```python
from build123d import *

# Parameters (mm, degrees)
F1_W         = 152.4
F1_H         = 101.6
F1_W_2       = 25.4
F1_H_2       = 25.4
F2_DEPTH     = 38.1
F3_W         = 153.4559056163
F3_H         = 102.0477414131
F3_W_2       = 152.4
F3_H_2       = 101.6
F4_DEPTH     = 0.508
F0_W         = 152.4
F0_H         = 101.6
F5_DEPTH     = 0.508
F6_T4_DEPTH  = 113.1193447297
F6_T9_DEPTH  = 113.1193447297
F6_T14_DEPTH = 113.1193447297


# Not quite as in the source:
# - a fillet or chamfer that OpenCascade refuses, or shapes differently, is made with other operations: its cross-section is extruded or revolved along the edge and cut away or added


with BuildPart() as f2:
    # F1 (on face) → F2 (new body)
    with BuildSketch(Plane.XY):
        Rectangle(F1_W, F1_H)
        with Locations((-36.918597445, -21.7081383014)):
            Rectangle(F1_W_2, F1_H_2, mode=Mode.SUBTRACT)
        with Locations((0, -21.855811876)):
            Rectangle(F1_W_2, F1_H_2, mode=Mode.SUBTRACT)
        with Locations((38.8383678732, -20.0837206056)):
            Rectangle(F1_W_2, F1_H_2, mode=Mode.SUBTRACT)
        with Locations((-41.6441853324, 23.0372088479)):
            Rectangle(F1_W_2, F1_H_2, mode=Mode.SUBTRACT)
        with Locations((0, 20.9697662408)):
            Rectangle(F1_W_2, F1_H_2, mode=Mode.SUBTRACT)
        with Locations((35.5895380648, 21.7081389993)):
            Rectangle(F1_W_2, F1_H_2, mode=Mode.SUBTRACT)
    extrude(amount=F2_DEPTH)

    # F3 (on face) → F4 (join)
    with BuildSketch(Plane.XY):
        with Locations((-0.3659911454, 0.1675821841)):
            Rectangle(F3_W, F3_H)
        Rectangle(F3_W_2, F3_H_2, mode=Mode.SUBTRACT)
    extrude(amount=F4_DEPTH)

    # F0 (on Top) → F5 (join)
    with BuildSketch(Plane.XY):
        Rectangle(F0_W, F0_H)
    extrude(amount=F5_DEPTH)

    # F6: fillet of radius 5.08 on 1 edges, made by hand


with BuildPart() as f6_tool2:
    # F6_s3 → F6_t4 (new body)
    with BuildSketch(Plane.XZ.offset(-56.7272545489)):
        with BuildLine():
            ThreePointArc((-74.8796232902, 0.508), (-76.0155458228, 0.3793715272), (-77.0939439535, 0))
            Line((-77.0939439535, 0), (-77.0939439535, 0.508))
            Line((-77.0939439535, 0.508), (-74.8796232902, 0.508))
        make_face()
    extrude(amount=F6_T4_DEPTH)

    split(bisect_by=Plane.XZ.offset(-50.8), keep=Keep.BOTTOM)


with BuildPart() as f2_1:
    add(f2.part)

    # F6_t1: cut F6_tool2
    add(f6_tool2.part, mode=Mode.SUBTRACT)


with BuildPart() as f6_tool7:
    # F6_s8 → F6_t9 (new body)
    with BuildSketch(Plane.XZ.offset(-56.7272545489)):
        with BuildLine():
            ThreePointArc((-74.8796232902, 0.508), (-76.0155458228, 0.3793715272), (-77.0939439535, 0))
            Line((-77.0939439535, 0), (-77.0939439535, 0.508))
            Line((-77.0939439535, 0.508), (-74.8796232902, 0.508))
        make_face()
    extrude(amount=F6_T9_DEPTH)

    split(bisect_by=Plane.YZ.offset(-76.2), keep=Keep.BOTTOM)


with BuildPart() as f2_2:
    add(f2_1.part)

    # F6_t6: cut F6_tool7
    add(f6_tool7.part, mode=Mode.SUBTRACT)


with BuildPart() as f6_tool12:
    # F6_s13 → F6_t14 (new body)
    with BuildSketch(Plane.XZ.offset(-56.7272545489)):
        with BuildLine():
            ThreePointArc((-74.8796232902, 0.508), (-76.0155458228, 0.3793715272), (-77.0939439535, 0))
            Line((-77.0939439535, 0), (-77.0939439535, 0.508))
            Line((-77.0939439535, 0.508), (-74.8796232902, 0.508))
        make_face()
    extrude(amount=F6_T14_DEPTH)

    split(bisect_by=Plane.XZ.offset(50.8), keep=Keep.TOP)


with BuildPart() as f2_3:
    add(f2_2.part)

    # F6_t11: cut F6_tool12
    add(f6_tool12.part, mode=Mode.SUBTRACT)


solid = f2_3.part
```
Verification items for the finished model (mm, model axes). A direction names the side the tool comes from. Round coordinates to 2 decimals unless told otherwise and drop trailing zeros. Loops run counter-clockwise (first coordinate to the right, second up) from the corner with the lowest first, then second, coordinate; pieces in that order, holes last. Notation, with made-up numbers: (-28, 16) -> (0, 16) arc R22 ccw to (0, 29) -> close; hole circle Ø6 at (52.5, -9). An arc over 180 degrees is marked (long way). Answer as a JSON object with one key per item and string values.
Q1. Draft check along X on faces 1 (the flat face through (-1, -50.8, 19)), 2 (the flat face through (26.138, -20, 19)), 3 (the flat face through (-76.2, -1, 19)), 4 (the flat face through (39, -32.784, 19)). Enter one of: pulls with the +X half, pulls with the -X half, needs draft (parallel to the pull), parting line crosses it, or undercut.
Data:
{"face 1": "needs draft", "face 2": "undercut", "face 3": "pulls with the -X half", "face 4": "undercut"}
Q2. Scan lines: line 1 (X direction, y = 24, z = 6.5); line 2 (X direction, y = -28.5, z = 33); line 3 (Y direction, x = 0, z = 28). Record each from-to range of solid material in increasing order. Write a range as from..to.
Data:
{"line 1": "x = -76.2..-54.34, -28.94..-12.7, 12.7..22.89, 48.29..76.2", "line 2": "x = -76.2..-49.62, -24.22..-12.7, 12.7..26.14, 51.54..76.2", "line 3": "y = -50.8..-34.56, -9.16..8.27, 33.67..50.8"}
Q3. Section check A-A (z = 24.5). Record the boundary of the cut face in (x, y), then the cut area to 3 significant figures.
Data:
{"outline": "(-76.2, -50.8) -> (76.2, -50.8) -> (76.2, 50.8) -> (-76.2, 50.8) -> close; hole (-54.34, 10.34) -> (-28.94, 10.34) -> (-28.94, 35.74) -> (-54.34, 35.74) -> close; hole (-49.62, -34.41) -> (-24.22, -34.41) -> (-24.22, -9.01) -> (-49.62, -9.01) -> close; hole (-12.7, -34.56) -> (12.7, -34.56) -> (12.7, -9.16) -> (-12.7, -9.16) -> close; hole (-12.7, 8.27) -> (12.7, 8.27) -> (12.7, 33.67) -> (-12.7, 33.67) -> close; hole (22.89, 9.01) -> (48.29, 9.01) -> (48.29, 34.41) -> (22.89, 34.41) -> close; hole (26.14, -32.78) -> (51.54, -32.78) -> (51.54, -7.38) -> (26.14, -7.38) -> close", "area": "11,600 mm2"}
Q4. Section check B-B (x = 4). Record the boundary of the cut face in (y, z).
Data:
{"outline": "(-50.86, 0) -> (51.19, 0) -> (51.19, 0.51) -> (50.8, 0.51) -> (50.8, 38.1) -> (33.67, 38.1) -> (33.67, 0.51) -> (8.27, 0.51) -> (8.27, 38.1) -> (-9.16, 38.1) -> (-9.16, 0.51) -> (-34.56, 0.51) -> (-34.56, 38.1) -> (-50.8, 38.1) -> (-50.8, 0.51) -> (-50.86, 0.51) -> close"}
Q5. Go/stop test with flat-tipped pins: P1, Ø11.5, axis at y = 1.5, z = 27, coming from the +X side; P2, Ø19, axis at x = 30, z = 22, coming from the -Y side; P3, Ø1.5, axis at y = -24, z = 14, coming from the -X side. Record where each tip stops, or that it passes through.
Data:
{"P1": "stops at x = 76.2", "P2": "stops at y = -50.8", "P3": "stops at x = -76.2"}
Q6. Access from +Z, -Z, +X, -X, +Y, -Y to the whole of each face (thin tool, end or side, straight path). Record for faces 5 (the flat face through (-1, 50.8, 19)), 6 (the flat face through (-37, -34.408, 19)).
Data:
{"face 5": "+Z, +X, -X, +Y", "face 6": "+Z"}
